Design review of the part built by this model. Coordinates are the model's own, in mm. A direction names the side the tool comes from. Coordinates: 2 decimals unless noted, no trailing zeros. Order: outer loops, then holes, each group sorted by start corner. A loop starts at its lowest first (then second) coordinate and runs counter-clockwise, first axis right, second up. Notation, with made-up numbers: M 36,56.5 L 75,56.5 A28 ccw 75,90.5 Z; hole C 10,40 d4. An arc over 180 degrees is marked long. Answer in a Markdown table with one row per item.
from build123d import *

# Parameters (mm, degrees)
SKETCH1_R           = 13.8
BOSS_EXTRUDE1_DEPTH = 40
SKETCH2_R           = 5
BOSS_EXTRUDE2_DEPTH = 3
SKETCH3_R           = 1
CUT_EXTRUDE1_DEPTH  = 3
SKETCH4_R           = 1.225
BOSS_EXTRUDE3_DEPTH = 3
FILLET1_R           = 1
FILLET2_R           = 0.5
SKETCH5_R           = 1.25
BOSS_EXTRUDE4_DEPTH = 6
FILLET3_R           = 0.2


with BuildPart() as part:
    # Sketch1 → Boss-Extrude1 (new body)
    with BuildSketch(Plane(origin=(0, 0, 0), x_dir=(1, 0, 0), z_dir=(0, 1, 0))):
        Circle(SKETCH1_R)
    extrude(amount=BOSS_EXTRUDE1_DEPTH)

    # Sketch2 → Boss-Extrude2 (add)
    with BuildSketch(Plane(origin=(0, 40, 0), x_dir=(1, 0, 0), z_dir=(0, 1, 0))):
        Circle(SKETCH2_R)
    extrude(amount=BOSS_EXTRUDE2_DEPTH)

    # Sketch3 → Cut-Extrude1 (cut)
    with BuildSketch(Plane(origin=(0, 40, 0), x_dir=(1, 0, 0), z_dir=(0, 1, 0))):
        with Locations((-8, 0)):
            Circle(SKETCH3_R)
        with Locations((8, 0)):
            Circle(SKETCH3_R)
    extrude(amount=-CUT_EXTRUDE1_DEPTH, mode=Mode.SUBTRACT)

    # Sketch4 → Boss-Extrude3 (add)
    with BuildSketch(Plane(origin=(0, 40, 0), x_dir=(1, 0, 0), z_dir=(0, 1, 0))):
        with Locations((0, 10.246950766)):
            Circle(SKETCH4_R)
    extrude(amount=BOSS_EXTRUDE3_DEPTH)

    # Fillet1
    fillet1_edges = [part.edges().sort_by_distance(p)[0] for p in [
        (-1.225, 43, -10.246950766),
    ]]
    fillet(fillet1_edges, radius=FILLET1_R)

    # Fillet2
    fillet2_edges = [part.edges().sort_by_distance(p)[0] for p in [
        (-13.8, 40, 0),
    ]]
    fillet(fillet2_edges, radius=FILLET2_R)

    # Sketch5 → Boss-Extrude4 (add)
    with BuildSketch(Plane(origin=(0, 43, 0), x_dir=(1, 0, 0), z_dir=(0, 1, 0))):
        Circle(SKETCH5_R)
    extrude(amount=BOSS_EXTRUDE4_DEPTH)

    # Fillet3
    fillet3_edges = [part.edges().sort_by_distance(p)[0] for p in [
        (-1.25, 49, 0),
    ]]
    fillet(fillet3_edges, radius=FILLET3_R)


solid = part.part
(1) Add section B-B, the plane y = 6. Give the boundary of the cut face in (x, z), and give its area (3 significant figures).
Return value:
| item | result |
|---|---|
| outline | C 0,0 d27.6 |
| area | 598 mm2 |
(2) Insertion check: pin 1 Ø1.8 at (x, z) = (8, 0) entering from +Y; pin 2 Ø1.6 at (x, z) = (8, 0.5) entering from +Y; pin 3 Ø4 at (x, y) = (-2.5, 24.5) entering from +Z. Each pin has a flat end and moves straight along its axis. Give the tip position at first contact, or say it passes through.
Return value:
| item | result |
|---|---|
| pin 1 | stops at y = 37 |
| pin 2 | stops at y = 40 |
| pin 3 | stops at z = 13.79 |
(3) For faces 1 (the flat face through (0, 49, 0)), 2 (the cylindrical face through (7.2, 38.5, 0.6)), list the 3-axis set-ups (+Z, -Z, +X, -X, +Y, -Y) from which the entire face can be reached by the end or side of a thin tool; tool diameter is ignored.
Return value:
| item | result |
|---|---|
| face 1 | +Z, -Z, +X, -X, +Y |
| face 2 | +Y |
(4) Draft analysis for pull direction Z (two halves, no side actions). For faces 3 (the flat face through (-8, 37, 0)), 4 (the flat face through (1, 43, 1)), 5 (the cylindrical face through (-1.796, 19.474, -13.683)), state which applies: pulls with the +Z half, pulls with the -Z half, needs draft (parallel to the pull), parting line crosses it, or undercut.
Return value:
| item | result |
|---|---|
| face 3 | undercut |
| face 4 | needs draft |
| face 5 | parting line crosses it |
(5) For line 1 along X through (y, z) = (38.05, 0); line 2 along Y through (x, z) = (11.5, -5.5); line 3 along Z through (x, y) = (8, 38.2), list the stretches that pass through material, from the lowest coordinate up. Write a range as from..to.
Return value:
| item | result |
|---|---|
| line 1 | x = -13.8..-9, -7..7, 9..13.8 |
| line 2 | y = 0..40 |
| line 3 | z = -11.24..-1, 1..11.24 |
(6) Add section A-A, the plane z = 0. Give the boundary of the cut face in (x, y), and give its area (3 significant figures).
Return value:
| item | result |
|---|---|
| outline | M -13.8,0 L 13.8,0 L 13.8,39.5 A0.5 ccw 13.3,40 L 9,40 L 9,37 L 7,37 L 7,40 L 5,40 L 5,43 L 1.25,43 L 1.25,48.8 A0.2 ccw 1.05,49 L -1.05,49 A0.2 ccw -1.25,48.8 L -1.25,43 L -5,43 L -5,40 L -7,40 L -7,37 L -9,37 L -9,40 L -13.3,40 A0.5 ccw -13.8,39.5 Z |
| area | 1,140 mm2 |
